from build123d import *

# Parameters (mm, degrees)
Y_KSEKLIK_EKSTR_ZYON1_DEPTH = 20
Y_KSEKLIK_EKSTR_ZYON2_DEPTH = 2
IZIM3_R                     = 2.5
KES_EKSTR_ZYON1_DEPTH       = 10


with BuildPart() as part:
    # Çizim1 → Yükseklik-Ekstrüzyon1 (new body)
    with BuildSketch(Plane.XY):
        with BuildLine():
            Line((-6.05, 0), (-6.05, -9))
            Line((-6.05, -9), (-16.05, -9))
            Line((-16.05, -9), (-16.05, -7))
            Line((-16.05, -7), (-8.05, -7))
            Line((-8.05, -7), (-8.05, 0))
            ThreePointArc((-8.05, 0), (0, 8.05), (8.05, 0))
            Line((8.05, 0), (8.05, -7))
            Line((8.05, -7), (16.05, -7))
            Line((16.05, -7), (16.05, -9))
            Line((16.05, -9), (6.05, -9))
            Line((6.05, -9), (6.05, 0))
            ThreePointArc((6.05, 0), (0, 6.05), (-6.05, 0))
        make_face()
    extrude(amount=Y_KSEKLIK_EKSTR_ZYON1_DEPTH)

    # Çizim2 → Yükseklik-Ekstrüzyon2 (add)
    with BuildSketch(Plane(origin=(0, -7, 0), x_dir=(1, 0, 0), z_dir=(0, 1, 0))):
        with BuildLine():
            Line((16.05, 0), (16.05, -20))
            ThreePointArc((16.05, -20), (26.05, -10), (16.05, 0))
        make_face()
    y_kseklik_ekstr_zyon2 = extrude(amount=-Y_KSEKLIK_EKSTR_ZYON2_DEPTH)

    # Aynalama1: Yükseklik-Ekstrüzyon2 across plane
    add(y_kseklik_ekstr_zyon2.mirror(Plane(origin=(0, 0, 0), x_dir=(0, 0, 1), z_dir=(1, 0, 0))))

    # Çizim3 → Kes-Ekstrüzyon1 (cut)
    with BuildSketch(Plane(origin=(0, -7, 0), x_dir=(1, 0, 0), z_dir=(0, 1, 0))):
        with Locations(Location((18.05, -10.202041029, 0), (0, 0, 270))):
            Circle(IZIM3_R)
        with Locations(Location((-18.05, -10.202041029, 0), (0, 0, 270))):
            Circle(IZIM3_R)
    extrude(amount=-KES_EKSTR_ZYON1_DEPTH, mode=Mode.SUBTRACT)


solid = part.part
The model under review builds one solid part; all positions refer to its coordinate system, in mm. A direction names the side the tool comes from. Coordinates: 2 decimals unless noted, no trailing zeros. Write each loop counter-clockwise with the first axis right and the second up, starting at its lowest first coordinate (ties: lowest second). Pieces come first, ordered by that corner, then holes. Notation, with made-up numbers: (-17.75, 58) - (30.25, 58) arc R20 ccw to (30.25, 76) - close; hole circle Ø7 at (18, 22). An arc over 180 degrees is marked (long way). Answer as a JSON object with one key per item and string values. Group by question number.
1. Add section B-B (x = -18.05). Give the boundary of the cut face in (y, z), plus the area to 3 significant figures.
2. Mouldability with a two-part tool opening along X and no side actions: class faces 4 (the face through (0.13, 6.05, 9.86)), 5 (the face through (7, -2, 0)), 6 (the face through (-8.05, -4, 10)) as pulls with the +X half, pulls with the -X half, needs draft (parallel to the pull), parting line crosses it, or undercut.
3. Add section D-D (z = 7). Give the boundary of the cut face in (x, y).
4. Add section C-C (z = 10). Give the boundary of the cut face in (x, y), plus the area to 3 significant figures.
5. Machinability: for faces 1 (the face through (-15, -7, 10)), 2 (the face through (8.05, -3, 10)), 3 (the face through (6.05, -5, 10)), which of the approach directions +Z, -Z, +X, -X, +Y, -Y give a long, thin tool a straight path to every point of the face, cutting with its end or side? Answer none if there is none.
6. Clearance check with flat-ended pins moving along their axes: pin 1 Ø4 at (x, z) = (-18.5, 11) entering from +Y; pin 2 Ø4.5 at (y, z) = (-3.5, 14) entering from +X; pin 3 Ø1 at (x, z) = (0.5, 14.5) entering from -Y. State where each tip first meets the part, or that it passes through.
7. To check wall thickness, follow probe 1 along X at (y, z) = (-4.5, 18.5); probe 2 along Y at (x, z) = (-24, 13.75); probe 3 along X at (y, z) = (2.25, 9.5). State the ranges of each line that lie inside material, in increasing order.
8. Add section A-A (y = -5). Give the boundary of the cut face in (x, z), plus the area to 3 significant figures.
Findings:
{
 "1": {"outline": "(-9, 0.2) - (-7, 0.2) - (-7, 7.7) - (-9, 7.7) - close; (-9, 12.7) - (-7, 12.7) - (-7, 19.8) - (-9, 19.8) - close", "area": "29.2 mm²"},
 "2": {"face 4": "undercut", "face 5": "needs draft", "face 6": "pulls with the -X half"},
 "3": {"outline": "(-25.59, -9) - (-6.05, -9) - (-6.05, 0) arc R6.05 cw to (6.05, 0) - (6.05, -9) - (25.59, -9) - (25.59, -7) - (8.05, -7) - (8.05, 0) arc R8.05 ccw to (-8.05, 0) - (-8.05, -7) - (-25.59, -7) - close"},
 "4": {"outline": "(-26.05, -9) - (-20.54, -9) - (-20.54, -7) - (-26.05, -7) - close; (-15.56, -9) - (-6.05, -9) - (-6.05, 0) arc R6.05 cw to (6.05, 0) - (6.05, -9) - (15.56, -9) - (15.56, -7) - (8.05, -7) - (8.05, 0) arc R8.05 ccw to (-8.05, 0) - (-8.05, -7) - (-15.56, -7) - close; (20.54, -9) - (26.05, -9) - (26.05, -7) - (20.54, -7) - close", "area": "132 mm²"},
 "5": {"face 1": "+Z, -Z, -X, +Y", "face 2": "+Z, -Z, +X, +Y", "face 3": "+Z, -Z, -Y"},
 "6": {"pin 1": "y = -7", "pin 2": "x = 8.05", "pin 3": "y = 5.97"},
 "7": {"probe 1": "-8.05 to -6.05, 6.05 to 8.05", "probe 2": "-9 to -7", "probe 3": "-7.73 to -5.62, 5.62 to 7.73"},
 "8": {"outline": "(-8.05, 0) - (-6.05, 0) - (-6.05, 20) - (-8.05, 20) - close; (6.05, 0) - (8.05, 0) - (8.05, 20) - (6.05, 20) - close", "area": "80.0 mm²"}
}
